For this review, use the dimensioned drawing (mm, ordinates from the lowest corner) and the shaded views. A direction names the side the tool comes from. Give positions to 0.01 mm unless a question says otherwise; leave off trailing zeros. Write each loop counter-clockwise with the first axis right and the second up, starting at its lowest first coordinate (ties: lowest second). Pieces come first, ordered by that corner, then holes. Notation, with made-up numbers: (36.25, 74) -> (62.25, 74) arc R21 cw to (62.25, 102) -> close; hole circle Ø8 at (47, 65). An arc over 180 degrees is marked (long way). Return JSON: item names as keys, results as strings.
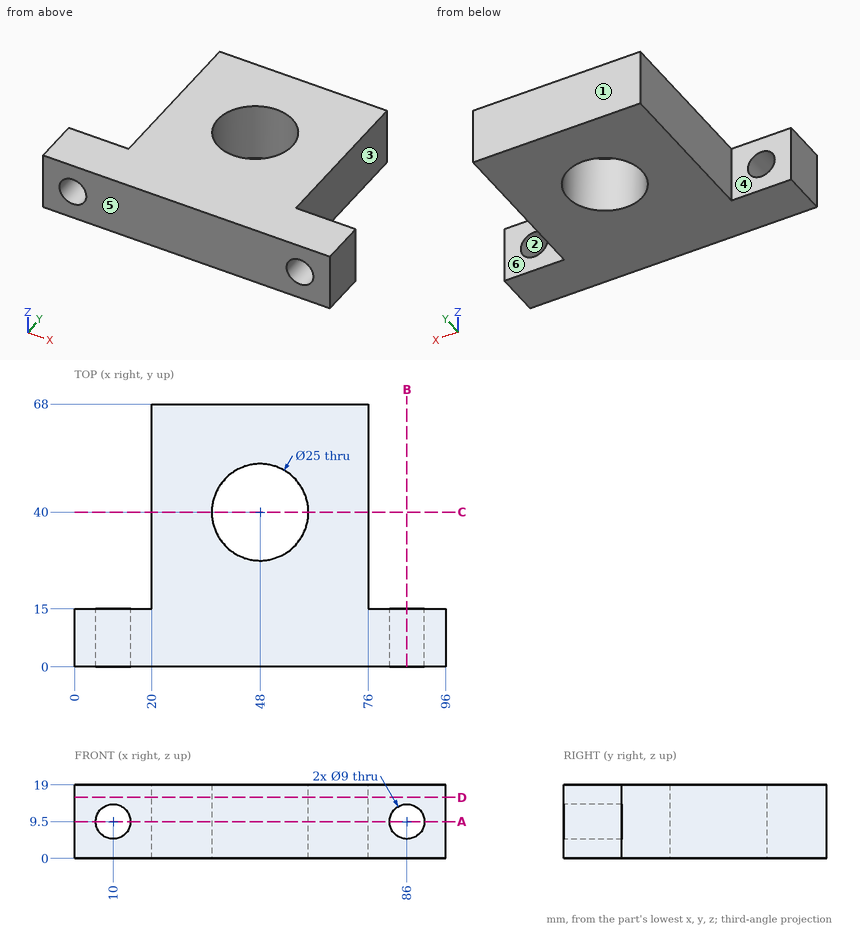
1. Add section A-A, the plane z = 9.5. State the section outline as (x, y) points.
Results found:
{"outline": "(0, 0) -> (5.5, 0) -> (5.5, 15) -> (0, 15) -> close; (14.5, 0) -> (81.5, 0) -> (81.5, 15) -> (76, 15) -> (76, 68) -> (20, 68) -> (20, 15) -> (14.5, 15) -> close; (90.5, 0) -> (96, 0) -> (96, 15) -> (90.5, 15) -> close; hole circle Ø25 at (48, 40)"}
2. Add section C-C, the plane y = 40. State the section outline as (x, z) points.
Results found:
{"outline": "(20, 0) -> (35.5, 0) -> (35.5, 19) -> (20, 19) -> close; (60.5, 0) -> (76, 0) -> (76, 19) -> (60.5, 19) -> close"}
3. To check wall thickness, follow probe 1 along X at (y, z) = (3.25, 9.5); probe 2 along X at (y, z) = (7, 13.25); probe 3 along Z at (x, y) = (86, 8.5). State the ranges of each line that lie inside material, in increasing order.
Results found:
{"probe 1": "x = 0 to 5.5, 14.5 to 81.5, 90.5 to 96", "probe 2": "x = 0 to 7.51, 12.49 to 83.51, 88.49 to 96", "probe 3": "z = 0 to 5, 14 to 19"}
4. Add section B-B, the plane x = 86. State the section outline as (y, z) points.
Results found:
{"outline": "(0, 0) -> (15, 0) -> (15, 5) -> (0, 5) -> close; (0, 14) -> (15, 14) -> (15, 19) -> (0, 19) -> close"}
5. The part is to be moulded in two halves that separate along X. For the marked faces 1, 2 and 3, say which applies: +X half, -X half, draft (parallel to the pull), parting line (faces both ways), or undercut.
Results found:
{"face 1": "draft", "face 2": "undercut", "face 3": "+X half"}
6. Add section D-D, the plane z = 15.75. State the section outline as (x, y) points.
Results found:
{"outline": "(0, 0) -> (96, 0) -> (96, 15) -> (76, 15) -> (76, 68) -> (20, 68) -> (20, 15) -> (0, 15) -> close; hole circle Ø25 at (48, 40)"}
7. For the marked faces 4, 5 and 6, list the 3-axis set-ups (+Z, -Z, +X, -X, +Y, -Y) from which the entire face can be reached by the end or side of a thin tool; tool diameter is ignored.
Results found:
{"face 4": "+Z, -Z, -X, +Y", "face 5": "+Z, -Z, +X, -X, -Y", "face 6": "+Z, -Z, +X, +Y"}
8. For pin 1 (6 mm diameter, centred on x = 85.5, z = 13.5, fed in from -Y); pin 2 (5 mm diameter, centred on x = 14.5, z = 7.5, fed in from +Y); pin 3 (9.5 mm diameter, centred on y = 32, z = 5, fed in from -X); pin 4 (1 mm diameter, centred on y = 52.5, z = 7.5, fed in from +X), all flat-tipped, find the tip position at first contact; note any pin that passes through.
Results found:
{"pin 1": "stops at y = 0", "pin 2": "stops at y = 15", "pin 3": "stops at x = 20", "pin 4": "stops at x = 76"}
